Work out the finished part from the listing and answer in its coordinate system (mm). Coordinates: 2 decimals unless noted, no trailing zeros. Write each loop counter-clockwise with the first axis right and the second up, starting at its lowest first coordinate (ties: lowest second). Pieces come first, ordered by that corner, then holes. Notation, with made-up numbers: (39, 51) - (63, 51) arc R25 cw to (63, 71) - close; hole circle Ø1 at (25, -31.5). An arc over 180 degrees is marked (long way). Answer as a JSON object with one key per item and string values. Group by question number.
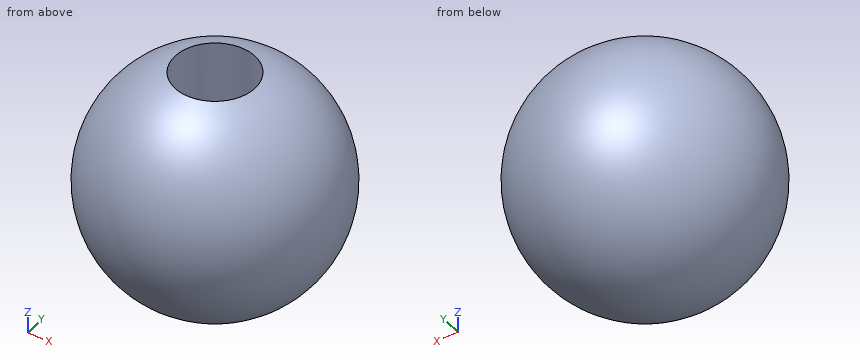
from build123d import *

# Parameters (mm, degrees)
F4_R     = 3.175
F5_DEPTH = 10.668
F6_DEPTH = 6.858


with BuildPart() as f2:
    # F0 (on Front) → F2 (revolve)
    with BuildSketch(Plane.XZ):
        with BuildLine():
            Line((0, -9.525), (0, 9.525))
            ThreePointArc((0, 9.525), (-9.525, 0), (0, -9.525))
        make_face()
    revolve(axis=Axis((0, 0, 0), (0, 0, 1)))

    # F4 (on offset) → F5 (cut)
    with BuildSketch(Plane.XY.offset(1.524)):
        Circle(F4_R)
    extrude(amount=F5_DEPTH, mode=Mode.SUBTRACT)

    # F4 (on offset) → F6 (cut)
    with BuildSketch(Plane.XY.offset(1.524)):
        Circle(F4_R)
    extrude(amount=F6_DEPTH, mode=Mode.SUBTRACT)


solid = f2.part
Q1. Section A-A on x = 0 is taken. Determine the outline of the cut face in (y, z) (3 decimals).
Q2. Flat-ended cylindrical pins translate along their axes: pin 1 Ø2 at (x, z) = (0, 5) entering from -Y; pin 2 Ø1 at (x, z) = (5.5, 2) entering from +Y; pin 3 Ø3 at (x, y) = (-0.5, -0.5) entering from +Z. Find the tip coordinate at first contact, or state that the pin passes through.
Q3. Section D-D on x = 5.5 is taken. Determine the outline of the cut face in (y, z).
Q4. Consider L1, parallel to X at y = 0, z = 7.5 (3 decimals); L2, parallel to Y at x = 0, z = 5.25 (3 decimals); L3, parallel to Y at x = 0, z = 4 (3 decimals). Determine where each line is inside the solid, lowest interval first. Write a range as from..to.
Q5. Section C-C on z = 3.25 is taken. Determine the outline of the cut face in (x, y) (3 decimals).
Numbers:
{
 "1": {"outline": "(-3.175, 1.524) - (-3.175, 8.98) arc R9.525 ccw (long way) to (3.175, 8.98) - (3.175, 1.524) - close"},
 "2": {"pin 1": "stops at y = -8.64", "pin 2": "stops at y = 7.88", "pin 3": "stops at z = 1.52"},
 "3": {"outline": "circle Ø15.55 at (0, 0)"},
 "4": {"L1": "x = -5.872..-3.175, 3.175..5.872", "L2": "y = -7.948..-3.175, 3.175..7.948", "L3": "y = -8.644..-3.175, 3.175..8.644"},
 "5": {"outline": "circle Ø17.907 at (0, 0); hole circle Ø6.35 at (0, 0)"}
}
